Job drawing, mm, ordinate dimensions from the low corner. One solid piece. A direction names the side the tool comes from. Coordinates: 2 decimals unless noted, no trailing zeros. Loops run counter-clockwise (first coordinate to the right, second up) from the corner with the lowest first, then second, coordinate; pieces in that order, holes last. Notation, with made-up numbers: (77.5, -12.75) - (135.5, -12.75) arc R4 ccw to (135.5, -8.75) - close; hole circle Ø1 at (85.25, 24.25). An arc over 180 degrees is marked (long way). Use a Markdown table: item, result. Add a question column.
1. Band-saw the part on C-C, the plane y = 5. Give the cut face in (x, z), plus the area to 3 significant figures.
2. Drop flat-ended pins along their axis: pin 1 (3 mm diameter, centred on x = 27.5, y = 9, fed in from -Z); pin 2 (4 mm diameter, centred on x = 7.5, z = 9, fed in from +Y); pin 3 (3.5 mm diameter, centred on x = 22, z = 4.5, fed in from -Y); pin 4 (1.8 mm diameter, centred on y = 30, z = 6.5, fed in from +X). Give the stop position or say it passes through.
3. Band-saw the part on D-D, the plane z = 9.5. Give the cut face in (x, y).
4. Wall check: probe 1 along Z at (x, y) = (31.95, 11); probe 2 along X at (y, z) = (3, 11.5); probe 3 along Z at (x, y) = (19.6, 2). Give the ranges that are in metal, low to high. Write a range as [from, to].
5. 3-axis set-ups, long thin cutter, end or side, ignore diameter. For the marked faces 1, 2, 3 and 4: which of +Z, -Z, +X, -X, +Y, -Y reach the whole face in a straight line?
6. Band-saw the part on A-A, the plane y = 30. Give the cut face in (x, z).
7. Band-saw the part on B-B, the plane x = 19.5. Give the cut face in (y, z), plus the area to 3 significant figures.
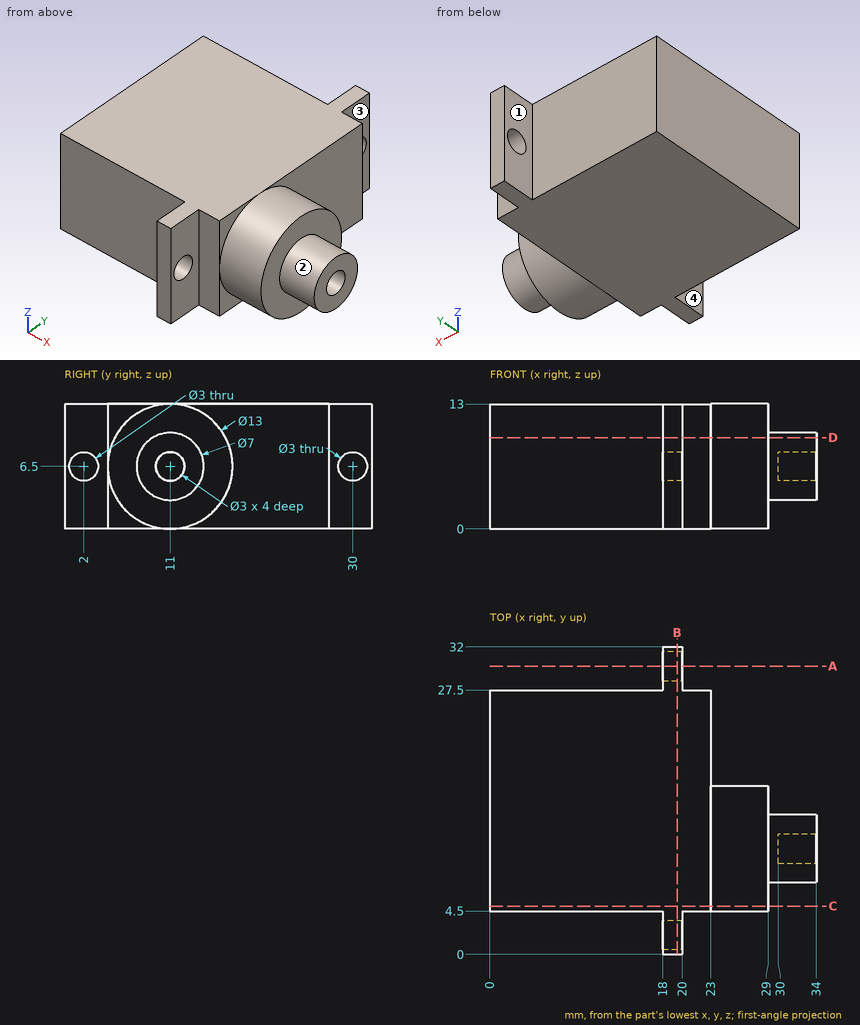
Geometry check:
| question | item | result |
|---|---|---|
| 1 | outline | (0, 0) - (23, 0) - (23, 4) - (29, 4) - (29, 9) - (23, 9) - (23, 13) - (0, 13) - close |
| 1 | area | 329 mm^2 |
| 2 | pin 1 | stops at z = 0.02 |
| 2 | pin 2 | stops at y = 27.5 |
| 2 | pin 3 | stops at y = 4.5 |
| 2 | pin 4 | passes through |
| 3 | outline | (0, 4.5) - (18, 4.5) - (18, 0) - (20, 0) - (20, 4.5) - (23, 4.5) - (23, 5.23) - (29, 5.23) - (29, 9.2) - (34, 9.2) - (34, 12.8) - (29, 12.8) - (29, 16.77) - (23, 16.77) - (23, 27.5) - (20, 27.5) - (20, 32) - (18, 32) - (18, 27.5) - (0, 27.5) - close |
| 4 | probe 1 | z = [3, 5], [8, 10] |
| 4 | probe 2 | x = [18, 20] |
| 4 | probe 3 | z = [0, 5], [8, 13] |
| 5 | face 1 | +Z, -Z, -X, +Y |
| 5 | face 2 | +X |
| 5 | face 3 | +Z, -Z, +X, +Y |
| 5 | face 4 | +Z, -Z, -X, -Y |
| 6 | outline | (18, 0) - (20, 0) - (20, 5) - (18, 5) - close; (18, 8) - (20, 8) - (20, 13) - (18, 13) - close |
| 7 | outline | (0, 0) - (32, 0) - (32, 13) - (0, 13) - close; hole circle Ø3 at (2, 6.5); hole circle Ø3 at (30, 6.5) |
| 7 | area | 402 mm^2 |
